from build123d import *

# Parameters (mm, degrees)
SKETCH4_W          = 800
SKETCH4_H          = 12
BASE_FLANGE1_DEPTH = 12
SKETCH9_W          = 10
SKETCH9_H          = 10
CUT_EXTRUDE2_DEPTH = 801.112492091
CUT_EXTRUDE3_DEPTH = 72


# Sheet-metal steps are written as plain solids
with BuildPart() as part:
    # Sketch4 → Base-Flange1 (new body)
    with BuildSketch(Plane(origin=(0, 0, 0), x_dir=(1, 0, 0), z_dir=(0, 1, 0))):
        Rectangle(SKETCH4_W, SKETCH4_H)
    extrude(amount=-BASE_FLANGE1_DEPTH)

    # Sketch9 → Cut-Extrude2 (cut, through all)
    with BuildSketch(Plane(origin=(400, 0, 0), x_dir=(0, 0, -1), z_dir=(1, 0, 0))):
        with Locations((0, -6)):
            Rectangle(SKETCH9_W, SKETCH9_H)
    extrude(amount=-CUT_EXTRUDE2_DEPTH, mode=Mode.SUBTRACT)

    # Sketch12 → Cut-Extrude3 (cut)
    with BuildSketch(Plane(origin=(0, 0, 0), x_dir=(1, 0, 0), z_dir=(0, 1, 0))):
        Polygon((-270, 5), (-281, -6), (-259, -6), align=None)
        Polygon((11, -6), (0, 5), (-11, -6), align=None)
        Polygon((141, -6), (130, 5), (119, -6), align=None)
        Polygon((-400, 6), (-388, -6), (-400, -6), align=None)
        Polygon((400, -6), (400, 6), (388, -6), align=None)
    extrude(amount=-CUT_EXTRUDE3_DEPTH, mode=Mode.SUBTRACT)


solid = part.part
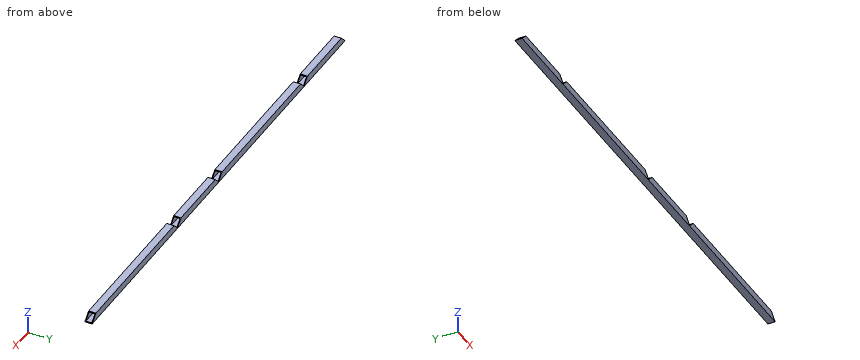
Input: part model. Units: mm. Frame: model coordinates. Coordinates: 2 decimals unless noted, no trailing zeros. Loops run counter-clockwise (first coordinate to the right, second up) from the corner with the lowest first, then second, coordinate; pieces in that order, holes last.
(1) Material intervals for probe 1 along Y at (x, z) = (-213, 1.5); probe 2 along Z at (x, y) = (-88, -7.75); probe 3 along X at (y, z) = (-11.5, 3.25), sorted ascending.
(2) Section A-A on z = 2.75. Count the separate pieces of the cut face and the enclosed holes in it, then the cut area to 3 significant figures.
(3) Section B-B on x = -47. Return the cut outline in (y, z), then the cut area to 3 significant figures.
(4) Section C-C on y = -3.25. Return the cut outline in (x, z).
(5) First-contact query: pin 1 Ø1.5 at (y, z) = (-10.5, 2.5) entering from -X; pin 2 Ø3 at (x, y) = (135.5, -7) entering from +Z. Flat tips, straight axial feed; report the tip coordinate or a pass-through.
Data:
1. probe 1: y = -12 to -11, -1 to 0
1. probe 2: z = -6 to -5, 5 to 6
1. probe 3: x = -390.75 to -278.25, -261.75 to -8.25, 8.25 to 121.75, 138.25 to 390.75
2. separate pieces: 8
2. enclosed holes: 0
2. area: 1,470 mm2
3. outline: (-12, -6) - (0, -6) - (0, 6) - (-12, 6) - close; hole (-11, -5) - (-1, -5) - (-1, 5) - (-11, 5) - close
3. area: 44.0 mm2
4. outline: (-400, -6) - (400, -6) - (399, -5) - (-399, -5) - close; (-389, 5) - (-280, 5) - (-281, 6) - (-388, 6) - close; (-260, 5) - (-10, 5) - (-11, 6) - (-259, 6) - close; (10, 5) - (120, 5) - (119, 6) - (11, 6) - close; (140, 5) - (389, 5) - (388, 6) - (141, 6) - close
5. pin 1: stops at x = -392.06
5. pin 2: stops at z = -5
